Design review of the part shown in the three views and the two pictorial views. Dimensions are in mm from the part's minimum x, y and z. A direction names the side the tool comes from. Give positions to 0.01 mm unless a question says otherwise; leave off trailing zeros. Order: outer loops, then holes, each group sorted by start corner. A loop starts at its lowest first (then second) coordinate and runs counter-clockwise, first axis right, second up.
Item 1: Machinability: for the marked faces 4 and 5, which of the approach directions +Z, -Z, +X, -X, +Y, -Y give a long, thin tool a straight path to every point of the face, cutting with its end or side? Answer none if there is none.
Item 2: Consider section A-A (y = 11.25). Give the boundary of the cut face in (x, z), plus the area to 3 significant figures.
Item 3: Consider section B-B (z = 43). Give the boundary of the cut face in (x, y), plus the area to 3 significant figures.
Item 4: Consider section C-C (x = 19). Give the boundary of the cut face in (y, z), plus the area to 3 significant figures.
Item 5: For P1, Ø4, axis at x = 8.5, y = 10, coming from the -Z side; P2, Ø3, axis at x = 8, z = 10, coming from the +Y side; P3, Ø2.5, axis at x = 17, z = 27, coming from the +Y side, all flat-tipped, find the tip position at first contact; note any pin that passes through.
Item 6: Consider section D-D (z = 23). Give the boundary of the cut face in (x, y).
Item 7: For probe 1 along Z at (x, y) = (19, 5.5); probe 2 along X at (y, z) = (7.25, 43); probe 3 along X at (y, z) = (10.25, 33), list the stretches that pass through material, from the lowest coordinate up.
Item 8: The part is to be moulded in two halves that separate along X. For the marked faces 1, 2 and 3, say which applies: released by +X, released by -X, zero draft, split by the parting line, or undercut.
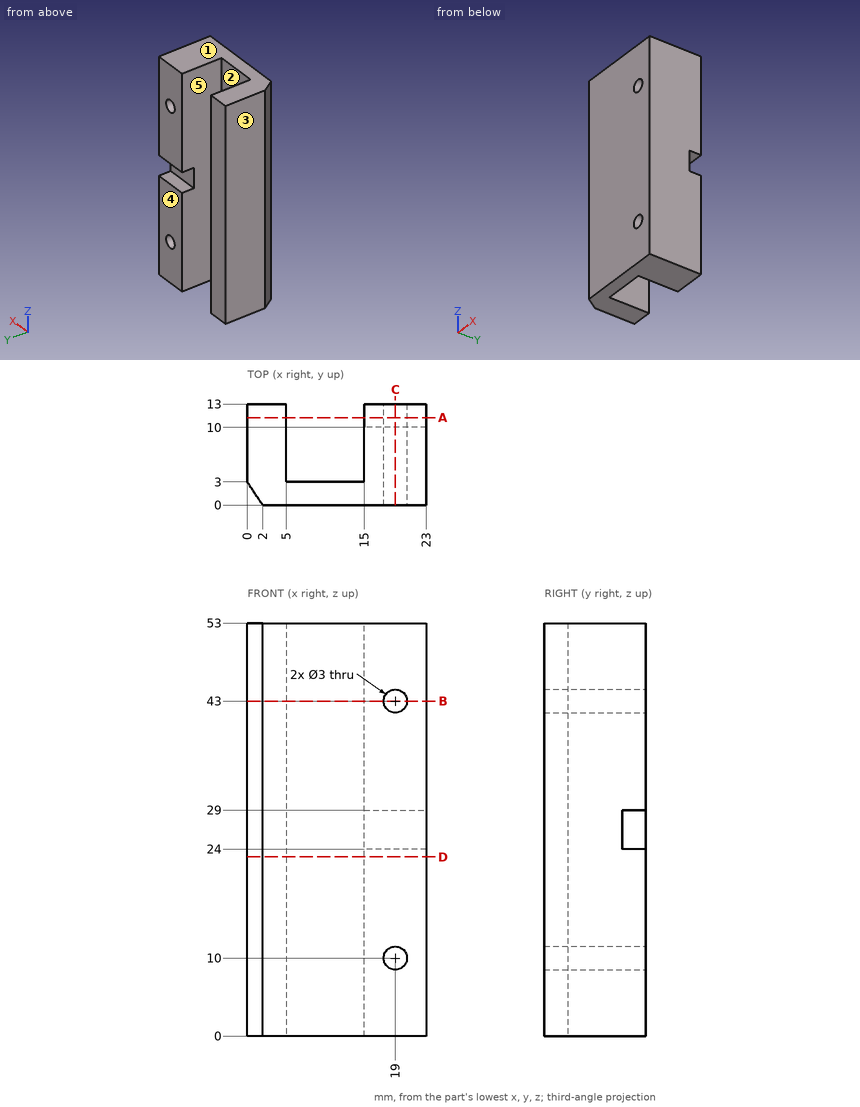
Resolved:
1. face 4: +Z, -Z, +X, -X, +Y
1. face 5: +Z, -Z, +Y
2. outline: (0, 0) - (5, 0) - (5, 53) - (0, 53) - close; (15, 0) - (23, 0) - (23, 24) - (15, 24) - close; (15, 29) - (23, 29) - (23, 53) - (15, 53) - close; hole circle Ø3 at (19, 10); hole circle Ø3 at (19, 43)
2. area: 635 mm2
3. outline: (0, 3) - (2, 0) - (17.5, 0) - (17.5, 13) - (15, 13) - (15, 3) - (5, 3) - (5, 13) - (0, 13) - close; (20.5, 0) - (23, 0) - (23, 13) - (20.5, 13) - close
3. area: 157 mm2
4. outline: (0, 0) - (13, 0) - (13, 8.5) - (0, 8.5) - close; (0, 11.5) - (13, 11.5) - (13, 24) - (10, 24) - (10, 29) - (13, 29) - (13, 41.5) - (0, 41.5) - close; (0, 44.5) - (13, 44.5) - (13, 53) - (0, 53) - close
4. area: 596 mm2
5. P1: passes through
5. P2: stops at y = 3
5. P3: stops at y = 10
6. outline: (0, 3) - (2, 0) - (23, 0) - (23, 13) - (15, 13) - (15, 3) - (5, 3) - (5, 13) - (0, 13) - close
7. probe 1: z = 0 to 8.5, 11.5 to 41.5, 44.5 to 53
7. probe 2: x = 0 to 5, 15 to 17.5, 20.5 to 23
7. probe 3: x = 0 to 5, 15 to 23
8. face 1: zero draft
8. face 2: undercut
8. face 3: released by -X
